Design review of the part built by this model. Coordinates are the model's own, in mm. A direction names the side the tool comes from. Coordinates: 2 decimals unless noted, no trailing zeros. Order: outer loops, then holes, each group sorted by start corner. A loop starts at its lowest first (then second) coordinate and runs counter-clockwise, first axis right, second up. Notation, with made-up numbers: M 66.5,-36.5 L 109.5,-36.5 A17 cw 109.5,-11.5 Z; hole C 38.25,28 d2. An arc over 180 degrees is marked long. Answer as a JSON object with one key per item and string values.
from build123d import *

# Parameters (mm, degrees)
SKETCH_R        = 27.5
PAD_DEPTH       = 8
POCKET_DEPTH    = 6
SKETCH013_R     = 1.75
POCKET006_DEPTH = 10
SKETCH021_W     = 35
SKETCH021_H     = 8
POCKET013_DEPTH = 2
SKETCH022_W     = 3
SKETCH022_H     = 5
POCKET014_DEPTH = 13


with BuildPart() as part:
    # Sketch → Pad (new body)
    with BuildSketch(Plane.XY):
        Circle(SKETCH_R)
    extrude(amount=PAD_DEPTH)

    # Sketch002 (on Face3 of Pad) → Pocket (cut)
    with BuildSketch(Plane.XY.offset(8)):
        Polygon((-18, 14), (-18, -14), (16.95, -14), (16.95, -12.3), (18, -11.25), (18, 6.25), (16.95, 7.3), (16.95, 14), align=None)
    extrude(amount=-POCKET_DEPTH, mode=Mode.SUBTRACT)

    # Sketch013 (on Face3 of Pocket) → Pocket006 (cut)
    with BuildSketch(Plane.XY.offset(8)):
        with Locations((-24, 0)):
            Circle(SKETCH013_R)
        with Locations((14.520833, 19.108778)):
            Circle(SKETCH013_R)
        with Locations((14.520833, -19.108778)):
            Circle(SKETCH013_R)
    extrude(amount=-POCKET006_DEPTH, mode=Mode.SUBTRACT)

    # Sketch021 (on Face15 of Pocket006) → Pocket013 (cut)
    with BuildSketch(Plane.XY.offset(2)):
        with Locations((-0.5, 9)):
            Rectangle(SKETCH021_W, SKETCH021_H)
        with Locations((-0.5, -9)):
            Rectangle(SKETCH021_W, SKETCH021_H)
    extrude(amount=-POCKET013_DEPTH, mode=Mode.SUBTRACT)

    # Sketch022 (on Face3 of Pocket013) → Pocket014 (cut)
    with BuildSketch(Plane.XY.offset(8)):
        with Locations((26, 0)):
            Rectangle(SKETCH022_W, SKETCH022_H)
    extrude(amount=-POCKET014_DEPTH, mode=Mode.SUBTRACT)


with BuildPart() as part_1:
    # Body placement: moved
    add(part.part.moved(Location((0, 0, 18))))


solid = part_1.part
1) Mouldability with a two-part tool opening along X and no side actions: class faces 5 (the flat face through (16.95, 11, 23)), 6 (the flat face through (0, 0, 18)), 7 (the cylindrical face through (-27.475, 1.174, 21.944)) as released by +X, released by -X, zero draft, split by the parting line, or undercut.
Taken from the geometry:
{"face 5": "undercut", "face 6": "zero draft", "face 7": "split by the parting line"}
2) Add section A-A (y = 0). State the section outline as (x, z) points.
Taken from the geometry:
{"outline": "M -27.5,18 L -25.75,18 L -25.75,26 L -27.5,26 Z; M -22.25,18 L 24.5,18 L 24.5,26 L 18,26 L 18,20 L -18,20 L -18,26 L -22.25,26 Z"}
3) Add section C-C (x = -24). State the section outline as (y, z) points.
Taken from the geometry:
{"outline": "M -13.43,18 L -1.75,18 L -1.75,26 L -13.43,26 Z; M 1.75,18 L 13.43,18 L 13.43,26 L 1.75,26 Z"}
4) Insertion check: pin 1 Ø1.6 at (y, z) = (-8, 19.5) entering from -X; pin 2 Ø0.5 at (x, y) = (1, 13.5) entering from +Z; pin 3 Ø1.8 at (x, z) = (1.5, 23.5) entering from +Y; pin 4 Ø3 at (x, y) = (14.52, -19.11) entering from +Z. Each pin has a flat end and moves straight along its axis. Give the tip position at first contact, or say it passes through.
Taken from the geometry:
{"pin 1": "stops at x = -26.54", "pin 2": "stops at z = 20", "pin 3": "stops at y = 27.49", "pin 4": "passes through"}
5) Add section D-D (z = 22.75). State the section outline as (x, y) points, and give its area (3 significant figures).
Taken from the geometry:
{"outline": "M 24.5,-2.5 L 24.5,2.5 L 27.39,2.5 A27.5 ccw long 27.39,-2.5 Z; hole C -24,0 d3.5; hole M -18,-14 L 16.95,-14 L 16.95,-12.3 L 18,-11.25 L 18,6.25 L 16.95,7.3 L 16.95,14 L -18,14 Z; hole C 14.52,-19.11 d3.5; hole C 14.52,19.11 d3.5", "area": "1,330 mm2"}
6) Tool access review of faces 1 (the flat face through (-1, -14, 23)), 2 (the flat face through (24.5, 0, 22)), 3 (the flat face through (-1, 5, 19)), 4 (the flat face through (17, 9, 19)): name each direction out of +Z, -Z, +X, -X, +Y, -Y from which nothing blocks a thin tool from reaching the whole face with its end or side.
Taken from the geometry:
{"face 1": "+Z", "face 2": "+Z, -Z, +X", "face 3": "+Z, -Z", "face 4": "-Z"}
7) Add section B-B (x = 0). State the section outline as (y, z) points.
Taken from the geometry:
{"outline": "M -27.5,18 L -13,18 L -13,20 L -14,20 L -14,26 L -27.5,26 Z; M -5,18 L 5,18 L 5,20 L -5,20 Z; M 13,18 L 27.5,18 L 27.5,26 L 14,26 L 14,20 L 13,20 Z"}
8) To check wall thickness, follow L1, parallel to Y at x = 15, z = 22.75; L2, parallel to Y at x = 16, z = 22; L3, parallel to Y at x = -2, z = 18.75. State the ranges of each line that lie inside material, in increasing order.
Taken from the geometry:
{"L1": "y = -23.05 to -20.79, -17.43 to -14, 14 to 17.43, 20.79 to 23.05", "L2": "y = -22.37 to -20.04, -18.17 to -14, 14 to 18.17, 20.04 to 22.37", "L3": "y = -27.43 to -13, -5 to 5, 13 to 27.43"}
